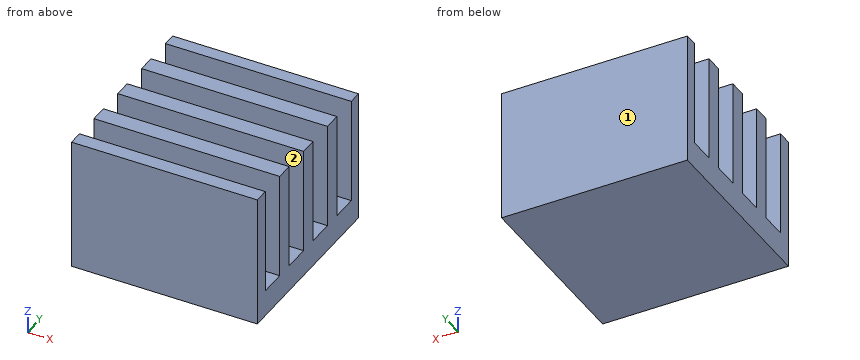
from build123d import *

# Parameters (mm, degrees)
SKETCH1_W           = 14
SKETCH1_H           = 14
BOSS_EXTRUDE1_DEPTH = 10
SKETCH2_W           = 8
SKETCH2_H           = 2
CUT_EXTRUDE1_DEPTH  = 15


with BuildPart() as part:
    # Sketch1 → Boss-Extrude1 (new body)
    with BuildSketch(Plane.XY):
        with Locations((23.5, 27.5)):
            Rectangle(SKETCH1_W, SKETCH1_H)
    extrude(amount=BOSS_EXTRUDE1_DEPTH)

    # Sketch2 → Cut-Extrude1 (cut, through all)
    with BuildSketch(Plane.ZY.offset(-16.5)):
        with Locations((6, 32.5)):
            Rectangle(SKETCH2_W, SKETCH2_H)
        with Locations((6, 29.2)):
            Rectangle(SKETCH2_W, SKETCH2_H)
        with Locations((6, 25.9)):
            Rectangle(SKETCH2_W, SKETCH2_H)
        with Locations((6, 22.6)):
            Rectangle(SKETCH2_W, SKETCH2_H)
    extrude(amount=-CUT_EXTRUDE1_DEPTH, mode=Mode.SUBTRACT)


solid = part.part
Source: CAD feature listing. Evaluate the final solid. Frame: model axes, mm. Face numbers are marked on the shaded views. A direction names the side the tool comes from. Coordinates: 2 decimals unless noted, no trailing zeros. Order: outer loops, then holes, each group sorted by start corner. A loop starts at its lowest first (then second) coordinate and runs counter-clockwise, first axis right, second up.
Item 1: Set-up query: the marked faces 1 and 2. Return all of +Z, -Z, +X, -X, +Y, -Y with unobstructed straight access to the full face (end or side cutting, diameter ignored); none if empty.
Output values:
face 1: +Z, -Z, +X, -X, +Y
face 2: +Z, +X, -X
Item 2: Material intervals for line 1 (Y direction, x = 17.75, z = 5.25); line 2 (Z direction, x = 27, y = 32.5), sorted ascending.
Output values:
line 1: y = 20.5 to 21.6, 23.6 to 24.9, 26.9 to 28.2, 30.2 to 31.5, 33.5 to 34.5
line 2: z = 0 to 2
Item 3: Cut plane B-B (x = 27.75). Return loops of the section in (y, z), plus the area to 3 significant figures.
Output values:
outline: (20.5, 0) - (34.5, 0) - (34.5, 10) - (33.5, 10) - (33.5, 2) - (31.5, 2) - (31.5, 10) - (30.2, 10) - (30.2, 2) - (28.2, 2) - (28.2, 10) - (26.9, 10) - (26.9, 2) - (24.9, 2) - (24.9, 10) - (23.6, 10) - (23.6, 2) - (21.6, 2) - (21.6, 10) - (20.5, 10) - close
area: 76.0 mm2
Item 4: Cut plane A-A (z = 6.5). Return loops of the section in (x, y), plus the area to 3 significant figures.
Output values:
outline: (16.5, 20.5) - (30.5, 20.5) - (30.5, 21.6) - (16.5, 21.6) - close; (16.5, 23.6) - (30.5, 23.6) - (30.5, 24.9) - (16.5, 24.9) - close; (16.5, 26.9) - (30.5, 26.9) - (30.5, 28.2) - (16.5, 28.2) - close; (16.5, 30.2) - (30.5, 30.2) - (30.5, 31.5) - (16.5, 31.5) - close; (16.5, 33.5) - (30.5, 33.5) - (30.5, 34.5) - (16.5, 34.5) - close
area: 84.0 mm2
Item 5: Cut plane C-C (y = 28.5). Return loops of the section in (x, z), plus the area to 3 significant figures.
Output values:
outline: (16.5, 0) - (30.5, 0) - (30.5, 2) - (16.5, 2) - close
area: 28.0 mm2
Item 6: First-contact query: P1, Ø5, axis at y = 22.5, z = 3.5, coming from the +X side. Flat tip, straight axial feed; report the tip coordinate or a pass-through.
Output values:
P1: stops at x = 30.5
